CAD build for the part. Positions are in the model's coordinates, mm. A direction names the side the tool comes from. Give positions to 0.01 mm unless a question says otherwise; leave off trailing zeros. Write each loop counter-clockwise with the first axis right and the second up, starting at its lowest first coordinate (ties: lowest second). Pieces come first, ordered by that corner, then holes. Notation, with made-up numbers: (1, -21) - (53, -21) arc R11 cw to (53, -4) - close; hole circle Ø6 at (8.5, -7.5). An arc over 180 degrees is marked (long way). Write item = value, one per line. Start each with the question number.
```python
from build123d import *


with BuildPart() as part:
    # 草圖1 → 旋轉1 (revolve)
    with BuildSketch(Plane.XY, mode=Mode.PRIVATE) as revolve_1_sk:
        Polygon((0, 0), (0, 19.795), (4.87, 19.795), (10.87, 10.213858447), (14.87, 10.213858447), (20.87, 19.795), (25.74, 19.795), (25.74, 10.213858447), (35.74, 10.213858447), (35.74, 0), align=None)
    revolve(revolve_1_sk.sketch.rotate(Axis((-743.15639781, 0, 0), (1, 0, 0)), 90), axis=Axis((-743.15639781, 0, 0), (1, 0, 0)))


solid = part.part
```
1. Tool access for faces 1 (the flat face through (25.74, 9, 9)), 2 (the cylindrical face through (12.9, -3.07, 9.74)), 3 (the cylindrical face through (23.339, -19.627, -2.577)): list every direction of +Z, -Z, +X, -X, +Y, -Y with a clear straight run to the whole face (end or side of a thin tool).
2. Wall check: line 1 along X through (y, z) = (5.5, -15); line 2 along X through (y, z) = (16.5, -10.5); line 3 along Y through (x, z) = (31.5, 0). Give the ranges that are in metal, low to high.
3. Cut at D-D (x = 3.5). Give the cut face in (y, z) (3 decimals), then the cut area to 3 significant figures.
4. Cut at C-C (x = 13). Give the cut face in (y, z).
5. Pin check, flat tips, straight feed: pin 1 Ø8 at (x, z) = (27, 7.5) entering from -Y; pin 2 Ø3 at (x, y) = (4, 6) entering from -Z; pin 3 Ø1 at (x, z) = (7, -10) entering from +Y. Stop position of each tip, or through.
6. Mould opens along X. For faces 4 (the cylindrical face through (2.469, -19.627, -2.577)), 5 (the conical face through (10.579, -10.588, -1.39)), 6 (the flat face through (0, 0, 0)) say: +X half, -X half, draft (parallel to the pull), parting line (faces both ways), or undercut.
7. Cut at A-A (y = 0). Give the cut face in (x, z) (3 decimals).
Output:
q1.face_1 = +X
q1.face_2 = none
q1.face_3 = +X, -X
q2.line_1 = 0 to 7.26, 18.48 to 25.74
q2.line_2 = 0 to 5.02, 20.72 to 25.74
q2.line_3 = -10.21 to 10.21
q3.outline = circle Ø39.59 at (0, 0)
q3.area = 1,230 mm2
q4.outline = circle Ø20.43 at (0, 0)
q5.pin_1 = -19.45
q5.pin_2 = -19.28
q5.pin_3 = 14.05
q6.face_4 = draft
q6.face_5 = undercut
q6.face_6 = -X half
q7.outline = (0, -19.795) - (4.87, -19.795) - (10.87, -10.214) - (14.87, -10.214) - (20.87, -19.795) - (25.74, -19.795) - (25.74, -10.214) - (35.74, -10.214) - (35.74, 10.214) - (25.74, 10.214) - (25.74, 19.795) - (20.87, 19.795) - (14.87, 10.214) - (10.87, 10.214) - (4.87, 19.795) - (0, 19.795) - close
